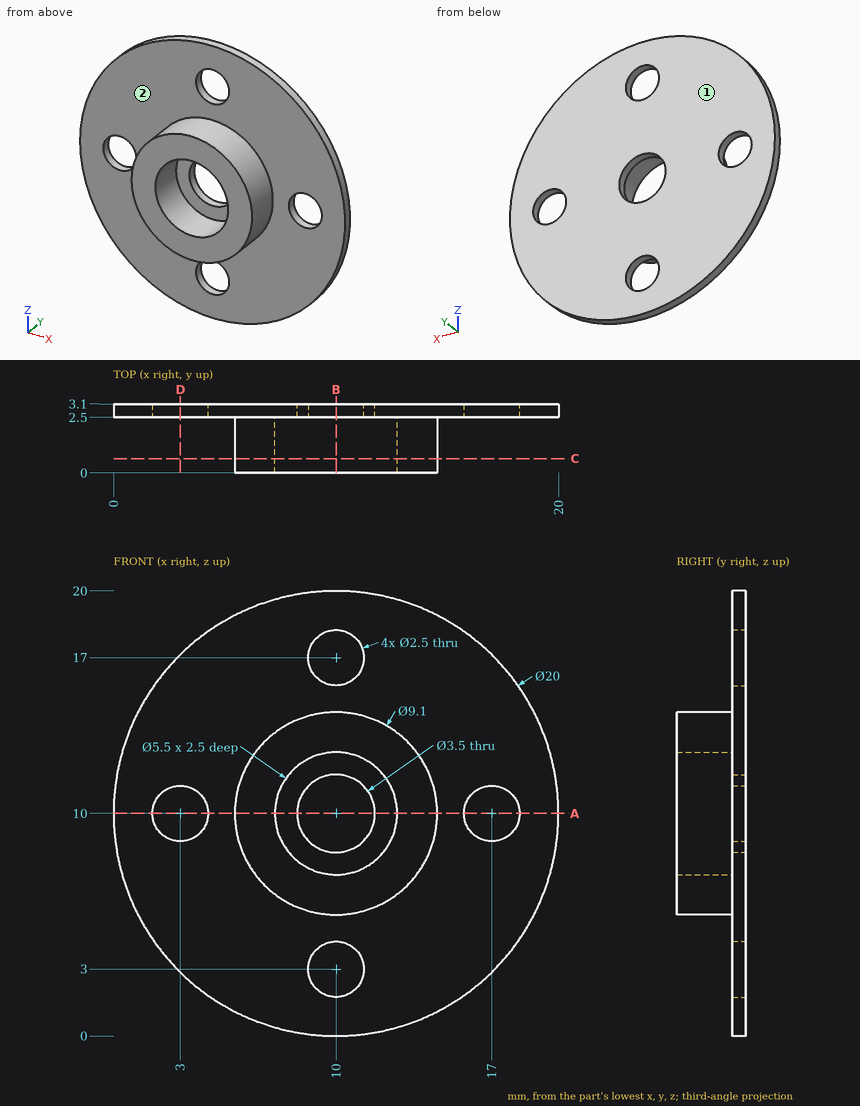
Part print with two shaded views. Sizes in mm from the minimum x, y, z corner. A direction names the side the tool comes from. Give positions to 0.01 mm unless a question says otherwise; leave off trailing zeros. Order: outer loops, then holes, each group sorted by start corner. A loop starts at its lowest first (then second) coordinate and runs counter-clockwise, first axis right, second up.
1) 3-axis set-ups, long thin cutter, end or side, ignore diameter. For the marked faces 1 and 2: which of +Z, -Z, +X, -X, +Y, -Y reach the whole face in a straight line?
2) Saw through at C-C, the plane y = 0.65. Write the cut outline in (x, z).
3) Wall check: probe 1 along Z at (x, y) = (10, 2.85); probe 2 along Z at (x, y) = (10, 1.25). Give the ranges that are in metal, low to high.
4) Saw through at A-A, the plane z = 10. Write the cut outline in (x, y), then the cut area to 3 significant figures.
5) Saw through at B-B, the plane x = 10. Write the cut outline in (y, z), then the cut area to 3 significant figures.
6) Pin check, flat tip, straight feed: pin 1 (4 mm diameter, centred on x = 10, z = 3, fed in from -Y). Stop position of the tip, or through.
7) Saw through at D-D, the plane x = 3. Write the cut outline in (y, z), then the cut area to 3 significant figures.
Computed:
1. face 1: +Z, -Z, +X, -X, +Y
1. face 2: -Y
2. outline: circle Ø9.1 at (10, 10); hole circle Ø5.5 at (10, 10)
3. probe 1: z = 0 to 1.75, 4.25 to 8.25, 11.75 to 15.75, 18.25 to 20
3. probe 2: z = 5.45 to 7.25, 12.75 to 14.55
4. outline: (0, 2.5) - (1.75, 2.5) - (1.75, 3.1) - (0, 3.1) - close; (4.25, 2.5) - (5.45, 2.5) - (5.45, 0) - (7.25, 0) - (7.25, 2.5) - (8.25, 2.5) - (8.25, 3.1) - (4.25, 3.1) - close; (11.75, 2.5) - (12.75, 2.5) - (12.75, 0) - (14.55, 0) - (14.55, 2.5) - (15.75, 2.5) - (15.75, 3.1) - (11.75, 3.1) - close; (18.25, 2.5) - (20, 2.5) - (20, 3.1) - (18.25, 3.1) - close
4. area: 15.9 mm2
5. outline: (0, 5.45) - (2.5, 5.45) - (2.5, 4.25) - (3.1, 4.25) - (3.1, 8.25) - (2.5, 8.25) - (2.5, 7.25) - (0, 7.25) - close; (0, 12.75) - (2.5, 12.75) - (2.5, 11.75) - (3.1, 11.75) - (3.1, 15.75) - (2.5, 15.75) - (2.5, 14.55) - (0, 14.55) - close; (2.5, 0) - (3.1, 0) - (3.1, 1.75) - (2.5, 1.75) - close; (2.5, 18.25) - (3.1, 18.25) - (3.1, 20) - (2.5, 20) - close
5. area: 15.9 mm2
6. pin 1: stops at y = 2.5
7. outline: (2.5, 2.86) - (3.1, 2.86) - (3.1, 8.75) - (2.5, 8.75) - close; (2.5, 11.25) - (3.1, 11.25) - (3.1, 17.14) - (2.5, 17.14) - close
7. area: 7.07 mm2
